from build123d import *

# Parameters (mm, degrees)
SKETCH1_R             = 35
SKETCH1_R_2           = 25
BOSS_EXTRUDE1_DEPTH   = 17.5
SKETCH5_R             = 5
BOSS_EXTRUDE3_DEPTH   = 10
BOSS_EXTRUDE3_2_DEPTH = 10
SKETCH4_R             = 5
BOSS_EXTRUDE5_DEPTH   = 10
BOSS_EXTRUDE5_2_DEPTH = 10
BOSS_EXTRUDE6_DEPTH   = 35
SKETCH14_R            = 5
BOSS_EXTRUDE12_DEPTH  = 5
BOSS_EXTRUDE13_DEPTH  = 35


with BuildPart() as part:
    # Sketch1 → Boss-Extrude1 (new body, symmetric)
    with BuildSketch(Plane(origin=(0, 0, 0), x_dir=(0, 0, -1), z_dir=(1, 0, 0))):
        Circle(SKETCH1_R)
        Circle(SKETCH1_R_2, mode=Mode.SUBTRACT)
    extrude(amount=BOSS_EXTRUDE1_DEPTH, both=True)



with BuildPart() as body_2:
    # Sketch5 → Boss-Extrude3 (new body)
    with BuildSketch(Plane.XY.offset(-7.5)):
        with BuildLine():
            Line((-17.5, -35), (-14.994489274, -127.40656046))
            ThreePointArc((-14.994489274, -127.40656046), (0, -142), (14.994489274, -127.40656046))
            Line((14.994489274, -127.40656046), (17.5, -35))
            Line((17.5, -35), (-17.5, -35))
        make_face()
        with Locations((0, -127)):
            Circle(SKETCH5_R, mode=Mode.SUBTRACT)
    extrude(amount=-BOSS_EXTRUDE3_DEPTH)


with BuildPart() as body_3:
    # Sketch5 → Boss-Extrude3 2 (new body)
    with BuildSketch(Plane.XY.offset(-7.5)):
        with BuildLine():
            Line((-17.5, 35), (17.5, 35))
            Line((17.5, 35), (51.609186621, 119.709648423))
            ThreePointArc((51.609186621, 119.709648423), (45.122886874, 140.458728374), (24.725687056, 132.938712227))
            Line((24.725687056, 132.938712227), (-17.5, 35))
        make_face()
        with Locations((38.5, 127)):
            Circle(SKETCH5_R, mode=Mode.SUBTRACT)
    extrude(amount=-BOSS_EXTRUDE3_2_DEPTH)


with BuildPart() as body_4:
    # Sketch4 → Boss-Extrude5 (new body)
    with BuildSketch(Plane.XY.offset(7.5)):
        with BuildLine():
            Line((-17.5, -35), (-14.994489274, -127.40656046))
            ThreePointArc((-14.994489274, -127.40656046), (0, -142), (14.994489274, -127.40656046))
            Line((14.994489274, -127.40656046), (17.5, -35))
            Line((17.5, -35), (-17.5, -35))
        make_face()
        with Locations((0, -127)):
            Circle(SKETCH4_R, mode=Mode.SUBTRACT)
    extrude(amount=BOSS_EXTRUDE5_DEPTH)


with BuildPart() as body_5:
    # Sketch4 → Boss-Extrude5 2 (new body)
    with BuildSketch(Plane.XY.offset(7.5)):
        with BuildLine():
            Line((-17.5, 35), (24.725687056, 132.938712227))
            ThreePointArc((24.725687056, 132.938712227), (45.122886874, 140.458728374), (51.609186621, 119.709648423))
            Line((51.609186621, 119.709648423), (17.5, 35))
            Line((17.5, 35), (-17.5, 35))
        make_face()
        with Locations((38.5, 127)):
            Circle(SKETCH4_R, mode=Mode.SUBTRACT)
    extrude(amount=BOSS_EXTRUDE5_2_DEPTH)


with BuildPart() as part_1:
    add(part.part)

    add(body_2.part)  # Boss-Extrude6 merges body 2

    add(body_3.part)  # Boss-Extrude6 merges body 3

    add(body_4.part)  # Boss-Extrude6 merges body 4

    add(body_5.part)  # Boss-Extrude6 merges body 5
    # Sketch7 → Boss-Extrude6 (add)
    with BuildSketch(Plane(origin=(17.5, 0, 0), x_dir=(0, 0, -1), z_dir=(1, 0, 0))):
        with BuildLine():
            Line((-17.5, 35), (-17.5, 30.310889132))
            ThreePointArc((-17.5, 30.310889132), (-12.64934905, 32.634245335), (-7.5, 34.186985828))
            Line((-7.5, 34.186985828), (-7.5, 35))
            Line((-7.5, 35), (-17.5, 35))
        make_face()
        with BuildLine():
            Line((7.5, 35), (7.5, 34.186985828))
            ThreePointArc((7.5, 34.186985828), (12.64934905, 32.634245335), (17.5, 30.310889132))
            Line((17.5, 30.310889132), (17.5, 35))
            Line((17.5, 35), (7.5, 35))
        make_face()
        with BuildLine():
            Line((7.5, -35), (7.5, -34.186985828))
            ThreePointArc((7.5, -34.186985828), (12.64934905, -32.634245335), (17.5, -30.310889132))
            Line((17.5, -30.310889132), (17.5, -35))
            Line((17.5, -35), (7.5, -35))
        make_face()
        with BuildLine():
            Line((-7.5, -35), (-7.5, -34.186985828))
            ThreePointArc((-7.5, -34.186985828), (-12.64934905, -32.634245335), (-17.5, -30.310889132))
            Line((-17.5, -30.310889132), (-17.5, -35))
            Line((-17.5, -35), (-7.5, -35))
        make_face()
    extrude(amount=-BOSS_EXTRUDE6_DEPTH)



with BuildPart() as body_2_2:
    # Sketch14 → Boss-Extrude12 (new body, symmetric)
    with BuildSketch(Plane(origin=(0, 0, 0), x_dir=(1, 0, 0), z_dir=(0, 1, 0))):
        with BuildLine():
            Line((17.5, -35), (31.392771581, -101.005420222))
            ThreePointArc((31.392771581, -101.005420222), (22.476413008, -115.632244571), (7.333133213, -107.624341112))
            Line((7.333133213, -107.624341112), (-17.5, -35))
            Line((-17.5, -35), (17.5, -35))
        make_face()
        with Locations((19.160783232, -103.58)):
            Circle(SKETCH14_R, mode=Mode.SUBTRACT)
        with Locations((9.580391616, -69.29)):
            Circle(SKETCH14_R, mode=Mode.SUBTRACT)
    extrude(amount=BOSS_EXTRUDE12_DEPTH, both=True)


with BuildPart() as part_2:
    add(part_1.part)

    add(body_2_2.part)  # Boss-Extrude13 merges body 2 2
    # Sketch15 → Boss-Extrude13 (add)
    with BuildSketch(Plane(origin=(17.5, 0, 0), x_dir=(0, 0, -1), z_dir=(1, 0, 0))):
        with BuildLine():
            Line((-35, 0), (-35, -5))
            Line((-35, -5), (-34.641016151, -5))
            ThreePointArc((-34.641016151, -5), (-34.91013868, -2.506435188), (-35, 0))
        make_face()
        with BuildLine():
            Line((-35, 5), (-35, 0))
            ThreePointArc((-35, 0), (-34.91013868, 2.506435188), (-34.641016151, 5))
            Line((-34.641016151, 5), (-35, 5))
        make_face()
    extrude(amount=-BOSS_EXTRUDE13_DEPTH)


solid = part_2.part
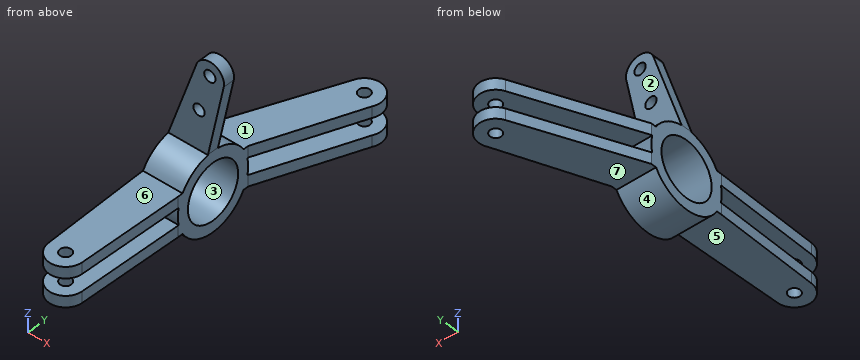
Geometry: final body of the model. Coordinates: model frame, mm. Face numbers are marked on the shaded views. A direction names the side the tool comes from. Round coordinates to 2 decimals unless told otherwise and drop trailing zeros. Loops run counter-clockwise (first coordinate to the right, second up) from the corner with the lowest first, then second, coordinate; pieces in that order, holes last. Notation, with made-up numbers: (74.25, 2.5) -> (107.25, 2.5) arc R17 ccw to (107.25, 20.5) -> close; hole circle Ø2 at (53, -8.5). An arc over 180 degrees is marked (long way). One line per question, with ' | ' between items. Start each with the question number.
1. Section D-D on y = 61. Output: boundary loops of the cut face in (x, z), and give its area (3 significant figures).
2. Contact query for flat-ended pins moving along their axis: pin 1 (1.5 mm diameter, centred on x = 5, y = -101.5, fed in from -Z); pin 2 (4 mm diameter, centred on y = -110, z = 14, fed in from +X); pin 3 (8 mm diameter, centred on x = 19.5, z = 31.5, fed in from +Y); pin 4 (8 mm diameter, centred on x = 0, y = -127, fed in from -Z). Output: stop coordinate, or through.
3. Mould query, pull axis Y, two halves, no side actions, for the marked faces 1, 2, 3 and 4. Classes: pulls with the +Y half, pulls with the -Y half, needs draft (parallel to the pull), parting line crosses it, or undercut.
4. Line query: line 1 along Z through (x, y) = (-1.5, -42); line 2 along Y through (x, z) = (-1, 0); line 3 along Y through (x, z) = (0, -10). Output: solid intervals per line, ascending. Write a range as [from, to].
5. Section A-A on y = 0. Output: boundary loops of the cut face in (x, z), and give its area (3 significant figures).
6. Set-up query: the marked faces 5, 6 and 7. Return all of +Z, -Z, +X, -X, +Y, -Y with unobstructed straight access to the full face (end or side cutting, diameter ignored); none if empty.
7. Section B-B on x = 10. Output: boundary loops of the cut face in (y, z), and give its area (3 significant figures).
8. Section C-C on z = 0. Output: boundary loops of the cut face in (x, y), and give its area (3 significant figures).
Returned:
1) outline: (-6.29, -17.5) -> (27.97, -17.5) -> (27.97, -7.5) -> (-6.29, -7.5) -> close; (-6.29, 7.5) -> (27.97, 7.5) -> (27.97, 17.5) -> (-6.29, 17.5) -> close | area: 685 mm2
2) pin 1: stops at z = -17.5 | pin 2: stops at x = 15.52 | pin 3: stops at y = 20.95 | pin 4: passes through
3) face 1: needs draft | face 2: pulls with the +Y half | face 3: undercut | face 4: parting line crosses it
4) line 1: z = [-17.5, -7.5], [7.5, 17.5] | line 2: y = [-35, -25], [25, 35] | line 3: y = [-142, -132], [-122, -22.91], [22.91, 75.59]
5) outline: (-17.5, -35) -> (17.5, -35) -> (17.5, -25) -> (-17.5, -25) -> close; (-17.5, 25) -> (17.5, 25) -> (17.5, 35) -> (31.39, 101.01) arc R12.5 ccw to (7.33, 107.62) -> (-17.5, 35) -> close; hole circle Ø10 at (9.58, 69.29); hole circle Ø10 at (19.16, 103.58) | area: 2,880 mm2
6) face 5: -Z, +X, -X, -Y | face 6: +Z, +X, -X, -Y | face 7: -Z, +X, -X, +Y
7) outline: (-138.18, -17.5) -> (-30.31, -17.5) arc R35 ccw to (30.31, -17.5) -> (98.78, -17.5) -> (98.78, -7.5) -> (34.19, -7.5) arc R35 ccw to (34.19, 7.5) -> (98.78, 7.5) -> (98.78, 17.5) -> (30.31, 17.5) arc R35 ccw to (5, 34.64) -> (5, 64.31) -> (-5, 64.31) -> (-5, 34.64) arc R35 ccw to (-30.31, 17.5) -> (-138.18, 17.5) -> (-138.18, 7.5) -> (-34.19, 7.5) arc R35 ccw to (-34.19, -7.5) -> (-138.18, -7.5) -> close; (-5, 74.27) -> (5, 74.27) -> (5, 112.08) -> (-5, 112.08) -> close; hole circle Ø50 at (0, 0) | area: 5,990 mm2
8) outline: (-17.5, -35) -> (17.5, -35) -> (17.5, -25) -> (-17.5, -25) -> close; (-17.5, 25) -> (17.5, 25) -> (17.5, 35) -> (-17.5, 35) -> close | area: 700 mm2
